Could you check a few things on this model? Use its own coordinates, in mm. Round coordinates to 2 decimals unless told otherwise and drop trailing zeros. Write each loop counter-clockwise with the first axis right and the second up, starting at its lowest first coordinate (ties: lowest second). Pieces come first, ordered by that corner, then holes. Notation, with made-up numbers: (-29, 12.25) -> (6, 12.25) arc R12 ccw to (6, 18.25) -> close; hole circle Ø4 at (-12, 27.5). An arc over 180 degrees is marked (long way). Answer in a Markdown table with one row per item.
from build123d import *

# Parameters (mm, degrees)
CONVERT_SOLID1_START     = -1.5
CONVERT_SOLID1_OUTLINE_R = 2.6
CONVERT_SOLID1_DEPTH     = 1.5


# Read off the part's stored shape, not the designer's step: Convert-Solid1
with BuildPart() as part:
    # Convert-Solid1 outline → Convert-Solid1 (new body)
    with BuildSketch(Plane.XY.offset(CONVERT_SOLID1_START)):
        with BuildLine():
            Line((15, 3), (15, 27))
            ThreePointArc((15, 27), (14.121320344, 29.121320344), (12, 30))
            Line((12, 30), (3, 30))
            ThreePointArc((3, 30), (0.878679656, 29.121320344), (0, 27))
            Line((0, 27), (0, 3))
            ThreePointArc((0, 3), (0.878679656, 0.878679656), (3, 0))
            Line((3, 0), (12, 0))
            ThreePointArc((12, 0), (14.121320344, 0.878679656), (15, 3))
        make_face()
        with Locations((7.5, 8)):
            Circle(CONVERT_SOLID1_OUTLINE_R, mode=Mode.SUBTRACT)
        with Locations((7.5, 22)):
            Circle(CONVERT_SOLID1_OUTLINE_R, mode=Mode.SUBTRACT)
    extrude(amount=CONVERT_SOLID1_DEPTH)


solid = part.part
1) Please list where these lines run through material, in increasing order: line 1 (Y direction, x = 7.5, z = -0.8); line 2 (Y direction, x = 9, z = -0.9); line 3 (X direction, y = 21, z = -1.05).
Findings:
| item | result |
|---|---|
| line 1 | y = 0 to 5.4, 10.6 to 19.4, 24.6 to 30 |
| line 2 | y = 0 to 5.88, 10.12 to 19.88, 24.12 to 30 |
| line 3 | x = 0 to 5.1, 9.9 to 15 |
2) Imagine slicing it at A-A, the plane x = 7.5. Please give me the cut outline in (y, z), plus the area to 3 significant figures.
Findings:
| item | result |
|---|---|
| outline | (0, -1.5) -> (5.4, -1.5) -> (5.4, 0) -> (0, 0) -> close; (10.6, -1.5) -> (19.4, -1.5) -> (19.4, 0) -> (10.6, 0) -> close; (24.6, -1.5) -> (30, -1.5) -> (30, 0) -> (24.6, 0) -> close |
| area | 29.4 mm^2 |
3) Imagine slicing it at B-B, the plane y = 22. Please give me the cut outline in (x, z).
Findings:
| item | result |
|---|---|
| outline | (0, -1.5) -> (4.9, -1.5) -> (4.9, 0) -> (0, 0) -> close; (10.1, -1.5) -> (15, -1.5) -> (15, 0) -> (10.1, 0) -> close |
4) Imagine slicing it at C-C, the plane z = -0.3. Please give me the cut outline in (x, y), plus the area to 3 significant figures.
Findings:
| item | result |
|---|---|
| outline | (0, 3) arc R3 ccw to (3, 0) -> (12, 0) arc R3 ccw to (15, 3) -> (15, 27) arc R3 ccw to (12, 30) -> (3, 30) arc R3 ccw to (0, 27) -> close; hole circle Ø5.2 at (7.5, 8); hole circle Ø5.2 at (7.5, 22) |
| area | 400 mm^2 |
5) Thinking about a two-plate mould opening in X: for faces 1 (the face through (14.1, 0.86, -0.76)), 2 (the face through (8.7, 5.693, -0.76)), 3 (the face through (7.162, 24.578, -0.76)), 4 (the face through (0.9, 29.14, -0.76)), which applies, +X half, -X half, draft (parallel to the pull), parting line (faces both ways), or undercut?
Findings:
| item | result |
|---|---|
| face 1 | +X half |
| face 2 | undercut |
| face 3 | undercut |
| face 4 | -X half |
6) For pin 1 (7 mm diameter, centred on x = 7.5, y = 22, fed in from +Z), with a flat end and sliding along its axis, tell me the tip position at first contact or that it passes through.
Findings:
| item | result |
|---|---|
| pin 1 | stops at z = 0 |
